The model under review builds one solid part; all positions refer to its coordinate system, in mm. A direction names the side the tool comes from. Give positions to 0.01 mm unless a question says otherwise; leave off trailing zeros. Loops run counter-clockwise (first coordinate to the right, second up) from the corner with the lowest first, then second, coordinate; pieces in that order, holes last. Notation, with made-up numbers: (22, 34.5) - (46, 34.5) arc R19 cw to (46, 68.5) - close; hole circle Ø11 at (-9, 5). An arc over 180 degrees is marked (long way). Return JSON: item names as keys, results as strings. Group by question number.
from build123d import *

# Parameters (mm, degrees)
F0_R     = 10.2235
F3_DEPTH = 5.715
F1_R     = 5.08
F4_DEPTH = 6.477
F2_R     = 4.064
F5_DEPTH = 9.779
F6_R     = 1.27


with BuildPart() as f3:
    # F0 (on Top) → F3 (new body)
    with BuildSketch(Plane.XY):
        Circle(F0_R)
    extrude(amount=F3_DEPTH)

    # F1 (on Top) → F4 (join)
    with BuildSketch(Plane.XY):
        Circle(F1_R)
    extrude(amount=F4_DEPTH)

    # F2 (on Top) → F5 (join)
    with BuildSketch(Plane.XY):
        Circle(F2_R)
    extrude(amount=F5_DEPTH)

    # F6
    f6_edges = [f3.edges().sort_by_distance(p)[0] for p in [
        (-10.2235, 0, 0),
    ]]
    fillet(f6_edges, radius=F6_R)


solid = f3.part
Item 1: For P1, Ø1.5, axis at y = -7, z = 1.5, coming from the -X side; P2, Ø4, axis at x = -3.5, y = 5, coming from the +Z side, all flat-tipped, find the tip position at first contact; note any pin that passes through.
Item 2: Take a section at C-C (z = 8.75). State the section outline as (x, y) points.
Item 3: Take a section at D-D (z = 4.25). State the section outline as (x, y) points.
Item 4: For L1, parallel to Z at x = -5.25, y = -7 (3 decimals); L2, parallel to Y at x = 4.5, z = 1.5; L3, parallel to X at y = -3, z = 1.75, list the stretches that pass through material, from the lowest coordinate up. Write a range as from..to.
Item 5: Tool access review of faces 1 (the face through (2, 5, 5.715)), 2 (the face through (0, 0, 0)): name each direction out of +Z, -Z, +X, -X, +Y, -Y from which nothing blocks a thin tool from reaching the whole face with its end or side.
Item 6: Take a section at A-A (x = 0). State the section outline as (y, z) points (1 decimal), then the cut area to 3 significant figures.
Check sheet entries:
{
 "1": {"P1": "stops at x = -8.09", "P2": "stops at z = 6.48"},
 "2": {"outline": "circle Ø8.13 at (0, 0)"},
 "3": {"outline": "circle Ø20.45 at (0, 0)"},
 "4": {"L1": "z = 0..5.715", "L2": "y = -9.18..9.18", "L3": "x = -9.77..9.77"},
 "5": {"face 1": "+Z", "face 2": "-Z, +X, -X, +Y, -Y"},
 "6": {"outline": "(-10.2, 1.3) arc R1.3 ccw to (-9, 0) - (9, 0) arc R1.3 ccw to (10.2, 1.3) - (10.2, 5.7) - (5.1, 5.7) - (5.1, 6.5) - (4.1, 6.5) - (4.1, 9.8) - (-4.1, 9.8) - (-4.1, 6.5) - (-5.1, 6.5) - (-5.1, 5.7) - (-10.2, 5.7) - close", "area": "151 mm^2"}
}
